```python
from build123d import *

# Parameters (mm, degrees)
F4_DEPTH = 3
F0_R     = 2.0664121369
F0_R_2   = 4
F0_R_3   = 14
F1_R     = 14
F1_R_2   = 14.6133175352
F1_R_3   = 4
F2_R     = 14
F5_DEPTH = 25


# Not quite as in the source:
# - ends of sketch curves that miss each other by under 0.0002 mm in the source are joined


with BuildPart() as f4:
    # F3 (on Top) → F4 (new body)
    with BuildSketch(Plane.XY):
        Polygon((1.2769951565, 200.9027954419), (1.2769951565, -215.7890487216), (10.8341440573, -225.3461976224), (12.7455411882, -227.2576774098), (12.7455411882, -232.9919504256), (50.9742194479, -232.9919504256), (50.9742194479, -227.2576774098), (79.6456661504, -227.2576774098), (79.6456661504, -232.9919504256), (117.8742627869, -232.9919504256), (117.8742627869, -227.2576774098), (146.5457921458, -227.2576774098), (146.5457921458, -232.9919504256), (184.774387749, -232.9919504256), (184.774387749, -227.2576774098), (184.774387749, 212.3715057533), (184.774387749, 218.1058614256), (146.5457921458, 218.1058614256), (146.5457921458, 212.3715057533), (117.8742627869, 212.3715057533), (117.8742627869, 218.1058614256), (79.6456661504, 218.1058614256), (79.6456661504, 212.3715057533), (50.9742194479, 212.3715057533), (50.9742194479, 218.1058614256), (12.7455411882, 218.1058614256), (12.7455411882, 212.3715057533), (10.8341440573, 210.4599443427), align=None)
    extrude(amount=F4_DEPTH)

    # F0 (on Top) + F1 (on Top) + F2 (on Top) → F5 (cut)
    with BuildSketch(Plane.XY):
        with Locations((30.7073234506, 204.3999841099)):
            Circle(F0_R)
        with Locations((70.0957699559, 203.6225220796)):
            Circle(F0_R_2)
        with Locations((115.556843684, 203.6225220796)):
            Circle(F0_R_2)
        with Locations((166.2479263408, 204.3999841099)):
            Circle(F0_R)
        with Locations((92.8263068199, 160.7444733381)):
            Circle(F0_R_3)
        with Locations((70.0957699559, 117.8664245966)):
            Circle(F0_R_2)
        with Locations((115.556843684, 117.8664245966)):
            Circle(F0_R_2)
        with Locations((30.5414876774, -218.1046205684)):
            Circle(F0_R)
        with Locations((166.247927374, -218.1046226348)):
            Circle(F0_R)
    with BuildSketch(Plane.XY):
        with Locations((106.8263068199, 93.8664245966)):
            Circle(F1_R)
        with Locations((68.3263068199, 86.8664245966)):
            Circle(F1_R)
        with Locations((92.8263068199, 60.8664245966)):
            Circle(F1_R_2)
        with Locations((98.8263068199, 24.8664245966)):
            Circle(F1_R)
        with Locations((54.3263068199, 53.8664245966)):
            Circle(F1_R)
        with Locations((60.3263068199, 18.3664245966)):
            Circle(F1_R)
        with Locations((107.0259951565, -131.3965302345)):
            Circle(F1_R)
        with Locations((68.5259951565, -138.3965302345)):
            Circle(F1_R)
        with Locations((54.5259951565, -171.3965302345)):
            Circle(F1_R)
        with Locations((93.0259951565, -164.3965302345)):
            Circle(F1_R_2)
        with Locations((99.0259951565, -200.3965302345)):
            Circle(F1_R)
        with Locations((60.5259951565, -206.8965302345)):
            Circle(F1_R)
        with Locations((92.0854285359, -64.518481493)):
            Circle(F1_R)
        with Locations((69.3548916719, -21.6404327515)):
            Circle(F1_R_3)
        with Locations((114.8159654, -21.6404327515)):
            Circle(F1_R_3)
        with Locations((114.8159654, -107.3965302345)):
            Circle(F1_R_3)
        with Locations((69.3548916719, -107.3965302345)):
            Circle(F1_R_3)
    with BuildSketch(Plane.XY):
        with Locations((21.9588205218, 41.3737557828)):
            Circle(F2_R)
        with Locations((21.9588422365, -56.2599998629)):
            Circle(F2_R)
    extrude(amount=F5_DEPTH, mode=Mode.SUBTRACT)


solid = f4.part
```
Input: part model. Units: mm. Frame: model coordinates. Give positions to 0.01 mm unless a question says otherwise; leave off trailing zeros. Write each loop counter-clockwise with the first axis right and the second up, starting at its lowest first coordinate (ties: lowest second). Pieces come first, ordered by that corner, then holes. Notation, with made-up numbers: (25, 19) - (74, 19) arc R27 ccw to (74, 42) - close; hole circle Ø4 at (24.5, 54). An arc over 180 degrees is marked (long way). Write item = value, one per line. Start each with the question number.
1. Section query A-A, the plane y = -56.26. Output: boundary loops of the cut face in (x, z).
2. Section query B-B, the plane x = 127. Output: boundary loops of the cut face in (y, z).
3. Ray query, L1, parallel to Y at x = 24.5, z = 1; L2, parallel to Y at x = 76, z = 2.25; L3, parallel to X at y = -151, z = 0.85. Return the intervals inside material, ascending.
4. Mould query, pull axis Y, two halves, no side actions, for faces 1 (the cylindrical face through (84.84, 25.48, 1.48)), 2 (the flat face through (92, -4, 0)). Classes: released by +Y, released by -Y, zero draft, split by the parting line, or undercut.
5. Section query C-C, the plane z = 2.5. Count the separate pieces of the cut face and the enclosed holes in it, then the cut area to 3 significant figures.
6. First-contact query: pin 1 Ø2.5 at (x, y) = (166.25, 204.4) entering from +Z; pin 2 Ø4 at (x, y) = (126.5, 163) entering from -Z; pin 3 Ø1.5 at (x, z) = (133.5, 1) entering from +Y. Flat tips, straight axial feed; report the tip coordinate or a pass-through.
Check sheet entries:
q1.outline = (1.28, 0) - (7.96, 0) - (7.96, 3) - (1.28, 3) - close; (35.96, 0) - (80.78, 0) - (80.78, 3) - (35.96, 3) - close; (103.39, 0) - (184.77, 0) - (184.77, 3) - (103.39, 3) - close
q2.outline = (-227.26, 0) - (212.37, 0) - (212.37, 3) - (-227.26, 3) - close
q3.L1 = -232.99 to -70.03, -42.49 to 27.61, 55.14 to 218.11
q3.L2 = -227.26 to -150.23, -126.56 to 75.16, 98.58 to 212.37
q3.L3 = 1.28 to 62.43, 74.62 to 87.19, 98.86 to 184.77
q4.face_1 = undercut
q4.face_2 = zero draft
q5.separate_pieces = 1
q5.enclosed_holes = 28
q5.area = 71,400 mm2
q6.pin_1 = through
q6.pin_2 = 0
q6.pin_3 = 212.37
